Drawing for the job (mm, zero at the part's lowest x, y, z). Coordinates: 2 decimals unless noted, no trailing zeros. Order: outer loops, then holes, each group sorted by start corner. A loop starts at its lowest first (then second) coordinate and runs counter-clockwise, first axis right, second up. Notation, with made-up numbers: (38.25, 29.5) -> (96.25, 29.5) arc R12 ccw to (96.25, 49.5) -> close; hole circle Ø9 at (51, -9). An arc over 180 degrees is marked (long way). Write each question's results on one line, items separated by ' | '.
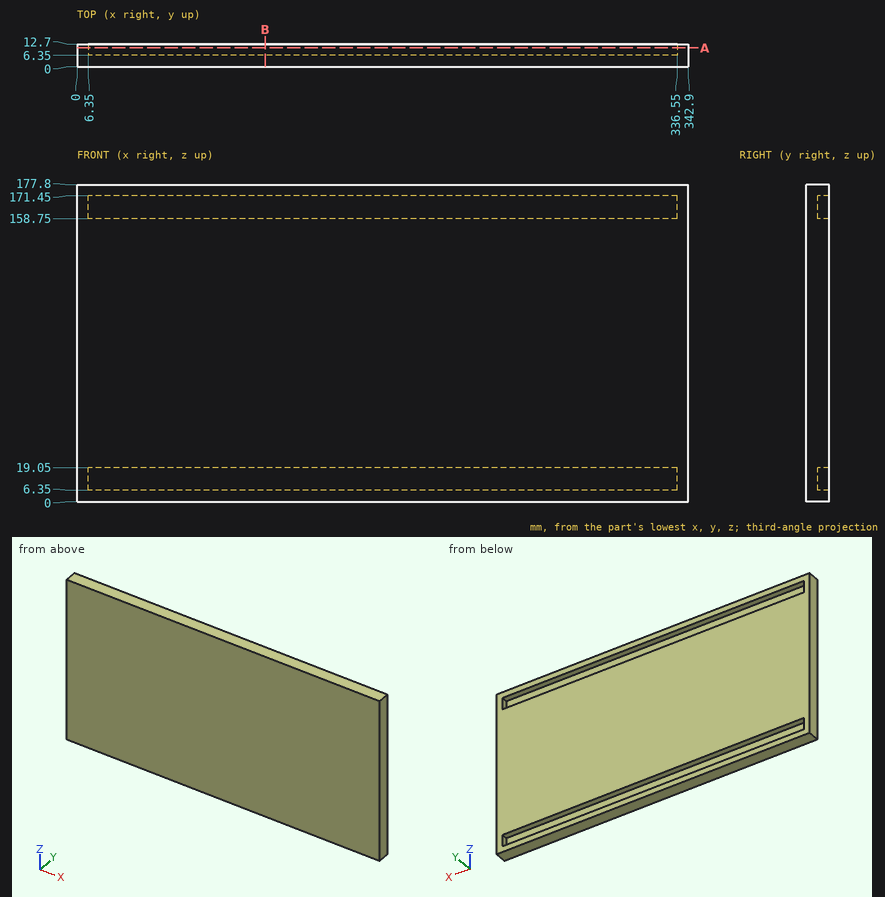
Item 1: Pin check, flat tip, straight feed: pin 1 (4 mm diameter, centred on x = 92, z = 166.5, fed in from +Y). Stop position of the tip, or through.
Answer:
pin 1: stops at y = 6.35
Item 2: Drill centre lines: line 1 (Z direction, x = 215, y = 8.5); line 2 (X direction, y = 12.25, z = 13); line 3 (Y direction, x = 236.5, z = 13.5). Where is each one in solid material? Low to high. Write a range as from..to.
Answer:
line 1: z = 0..6.35, 19.05..158.75, 171.45..177.8 | line 2: x = 0..6.35, 336.55..342.9 | line 3: y = 0..6.35
Item 3: Slice it at B-B, the plane x = 105.5. List the corners of the cut face in (y, z).
Answer:
outline: (0, 0) -> (12.7, 0) -> (12.7, 6.35) -> (6.35, 6.35) -> (6.35, 19.05) -> (12.7, 19.05) -> (12.7, 158.75) -> (6.35, 158.75) -> (6.35, 171.45) -> (12.7, 171.45) -> (12.7, 177.8) -> (0, 177.8) -> close
Item 4: Slice it at A-A, the plane y = 10.5. List the corners of the cut face in (x, z).
Answer:
outline: (0, 0) -> (342.9, 0) -> (342.9, 177.8) -> (0, 177.8) -> close; hole (6.35, 6.35) -> (336.55, 6.35) -> (336.55, 19.05) -> (6.35, 19.05) -> close; hole (6.35, 158.75) -> (336.55, 158.75) -> (336.55, 171.45) -> (6.35, 171.45) -> close
